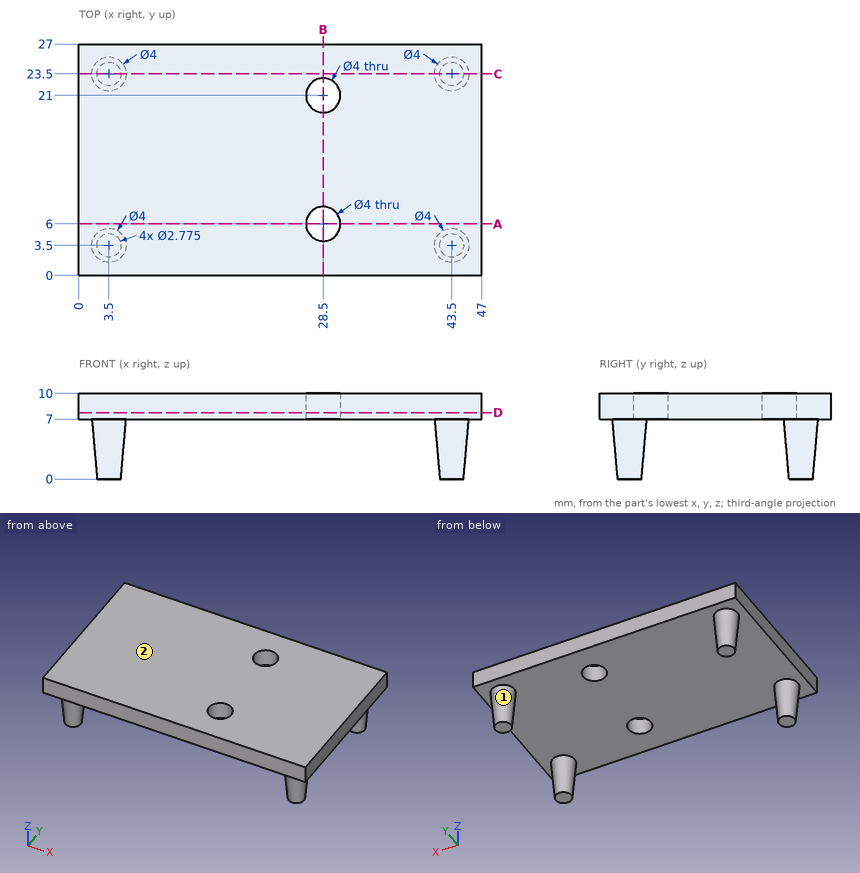
Part print with two shaded views. Sizes in mm from the minimum x, y, z corner. Give positions to 0.01 mm unless a question says otherwise; leave off trailing zeros. Write each loop counter-clockwise with the first axis right and the second up, starting at its lowest first coordinate (ties: lowest second). Pieces come first, ordered by that corner, then holes.
1) Cut at A-A on y = 6. Write the cut outline in (x, z), then the cut area to 3 significant figures.
Resolved:
outline: (0, 7) - (26.5, 7) - (26.5, 10) - (0, 10) - close; (30.5, 7) - (47, 7) - (47, 10) - (30.5, 10) - close
area: 129 mm2
2) Cut at B-B on x = 28.5. Write the cut outline in (y, z).
Resolved:
outline: (0, 7) - (4, 7) - (4, 10) - (0, 10) - close; (8, 7) - (19, 7) - (19, 10) - (8, 10) - close; (23, 7) - (27, 7) - (27, 10) - (23, 10) - close
3) Two-plate mould, pull along X, no slides. Class the marked faces 1 and 2: released by +X, released by -X, zero draft, split by the parting line, or undercut.
Resolved:
face 1: undercut
face 2: zero draft
4) Pin check, flat tips, straight feed: pin 1 (3 mm diameter, centred on y = 8.5, z = 1.5, fed in from +X); pin 2 (4.5 mm diameter, centred on x = 28.5, y = 6, fed in from -Z). Stop position of each tip, or through.
Resolved:
pin 1: passes through
pin 2: stops at z = 7
5) Probe L1, parallel to Y at x = 28.5, z = 8.85; L2, parallel to Z at x = 36, y = 9; L3, parallel to X at y = 23, z = 6.5. List the from-to ranges inside material, lowest first.
Resolved:
L1: y = 0 to 4, 8 to 19, 23 to 27
L2: z = 7 to 10
L3: x = 1.61 to 5.39, 41.61 to 45.39
6) Cut at D-D on z = 7.75. Write the cut outline in (x, y), then the cut area to 3 significant figures.
Resolved:
outline: (0, 0) - (47, 0) - (47, 27) - (0, 27) - close; hole circle Ø4 at (28.5, 6); hole circle Ø4 at (28.5, 21)
area: 1,240 mm2
7) Cut at C-C on y = 23.5. Write the cut outline in (x, z), then the cut area to 3 significant figures.
Resolved:
outline: (0, 7) - (1.5, 7) - (2.11, 0) - (4.89, 0) - (5.5, 7) - (41.5, 7) - (42.11, 0) - (44.89, 0) - (45.5, 7) - (47, 7) - (47, 10) - (0, 10) - close
area: 188 mm2
